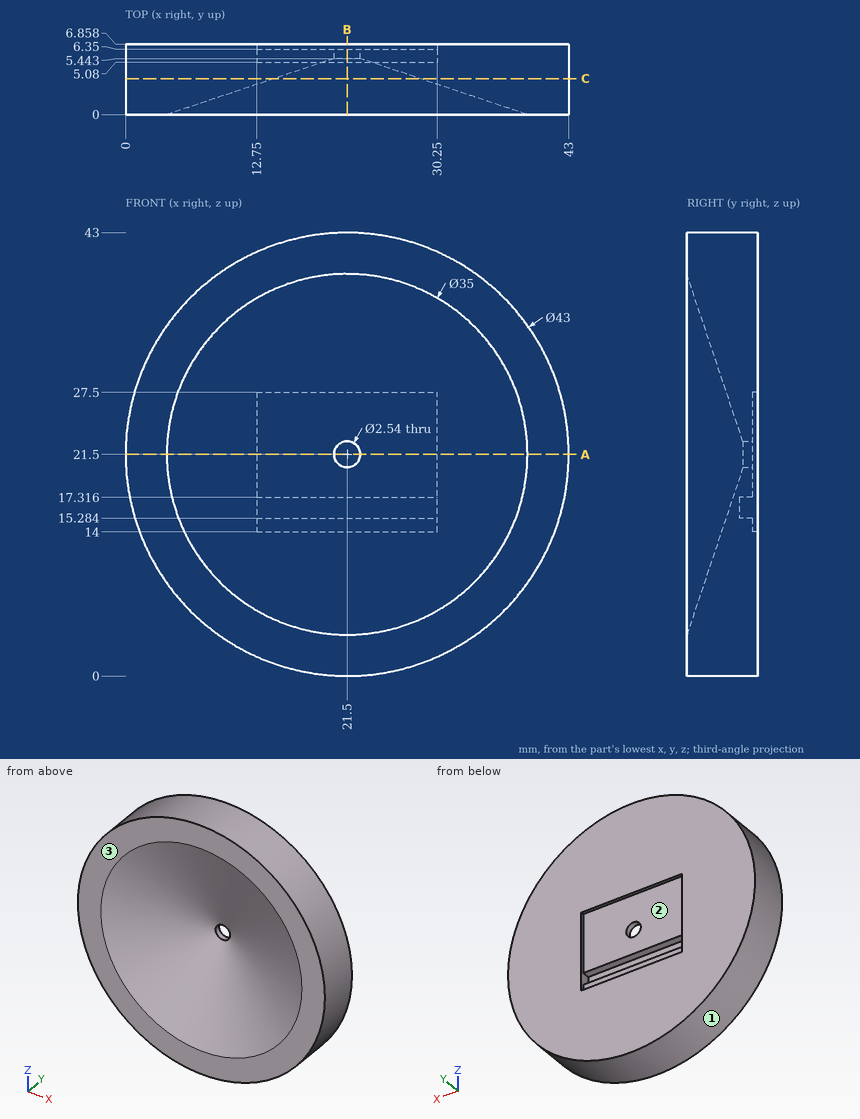
Job drawing, mm, ordinate dimensions from the low corner. One solid piece. Coordinates: 2 decimals unless noted, no trailing zeros. Order: outer loops, then holes, each group sorted by start corner. A loop starts at its lowest first (then second) coordinate and runs counter-clockwise, first axis right, second up. Notation, with made-up numbers: (-19.5, 4.5) - (13.5, 4.5) arc R9 cw to (13.5, 13.5) - close; hole circle Ø11 at (-34.75, -13). An arc over 180 degrees is marked (long way). Return JSON: item names as keys, results as strings. Group by question number.
1) Saw through at A-A, the plane z = 21.5. Write the cut outline in (x, y).
2) Saw through at B-B, the plane x = 21.5. Write the cut outline in (y, z), plus the area to 3 significant figures.
3) Mould opens along X. For the marked faces 1, 2 and 3 say: released by +X, released by -X, zero draft, split by the parting line, or undercut.
4) Probe line 1 (Z direction, x = 21.5, y = 6.1); line 2 (X direction, y = 4.75, z = 34); line 3 (Z direction, x = 16, y = 6.25) (1 decimal). List the from-to ranges inside material, lowest first. Write a range as from..to.
5) Flat gauge pins, fed straight in: P1, Ø4, axis at x = 11.5, y = 2.5, coming from the +Z side; P2, Ø1, axis at x = 6, y = 3, coming from the +Z side; P3, Ø0.5, axis at y = 6, z = 23, coming from the +X side; P4, Ø1.5, axis at x = 21.5, z = 21.5, coming from the +Y side. Where does each tip first touch, or does it go through?
6) Saw through at C-C, the plane y = 3.5. Write the cut outline in (x, z).
Values found:
{
 "1": {"outline": "(0, 0) - (4, 0) - (20.23, 5.44) - (20.23, 6.35) - (12.75, 6.35) - (12.75, 6.86) - (0, 6.86) - close; (22.77, 5.44) - (39, 0) - (43, 0) - (43, 6.86) - (30.25, 6.86) - (30.25, 6.35) - (22.77, 6.35) - close"},
 "2": {"outline": "(0, 0) - (6.86, 0) - (6.86, 14) - (6.35, 14) - (6.35, 15.28) - (5.08, 15.28) - (5.08, 17.32) - (6.35, 17.32) - (6.35, 20.23) - (5.44, 20.23) - (0, 4) - close; (0, 39) - (5.44, 22.77) - (6.35, 22.77) - (6.35, 27.5) - (6.86, 27.5) - (6.86, 43) - (0, 43) - close", "area": "181 mm²"},
 "3": {"face 1": "split by the parting line", "face 2": "undercut", "face 3": "zero draft"},
 "4": {"line 1": "z = 0..15.28, 17.32..20.23, 22.77..43", "line 2": "x = 4.01..38.99", "line 3": "z = 0.7..15.3, 17.3..42.3"},
 "5": {"P1": "stops at z = 41.46", "P2": "stops at z = 36.9", "P3": "stops at x = 42.96", "P4": "passes through"},
 "6": {"outline": "circle Ø43 at (21.5, 21.5); hole circle Ø14.13 at (21.5, 21.5)"}
}
